```python
from build123d import *

# Parameters (mm, degrees)
SKETCH1_W           = 25
SKETCH1_H           = 50
BOSS_EXTRUDE1_DEPTH = 4.5
CUT_EXTRUDE1_DEPTH  = 4.5
LPATTERN1_COUNT     = 2
LPATTERN1_PITCH     = 16
CUT_EXTRUDE2_REACH  = 6.5


with BuildPart() as part:
    # Sketch1 → Boss-Extrude1 (new body)
    with BuildSketch(Plane.XY):
        with Locations((12.5, 25)):
            Rectangle(SKETCH1_W, SKETCH1_H)
    extrude(amount=BOSS_EXTRUDE1_DEPTH)

    # Sketch2 → Cut-Extrude1 (cut)
    with BuildSketch(Plane.XY.offset(4.5)):
        with BuildLine():
            Line((12.5, 10.25), (14.25, 10.25))
            ThreePointArc((14.25, 10.25), (14.636370331, 9.953527618), (14.45, 9.503589838))
            ThreePointArc((14.45, 9.503589838), (14.303589838, 9.357179677), (14.25, 9.157179677))
            Line((14.25, 9.157179677), (14.25, 8))
            Line((14.25, 8), (14.25, 6.842820323))
            ThreePointArc((14.25, 6.842820323), (14.303589838, 6.642820323), (14.45, 6.496410162))
            ThreePointArc((14.45, 6.496410162), (14.636370331, 6.046472382), (14.25, 5.75))
            Line((14.25, 5.75), (12.5, 5.75))
            Line((12.5, 5.75), (10.75, 5.75))
            ThreePointArc((10.75, 5.75), (10.363629669, 6.046472382), (10.55, 6.496410162))
            ThreePointArc((10.55, 6.496410162), (10.696410162, 6.642820323), (10.75, 6.842820323))
            Line((10.75, 6.842820323), (10.75, 8))
            Line((10.75, 8), (10.75, 9.157179677))
            ThreePointArc((10.75, 9.157179677), (10.696410162, 9.357179677), (10.55, 9.503589838))
            ThreePointArc((10.55, 9.503589838), (10.363629669, 9.953527618), (10.75, 10.25))
            Line((10.75, 10.25), (12.5, 10.25))
        make_face()
    cut_extrude1 = extrude(amount=-CUT_EXTRUDE1_DEPTH, mode=Mode.SUBTRACT)

    # LPattern1: Cut-Extrude1 ×2
    with Locations(*[(0, i * LPATTERN1_PITCH, 0) for i in range(1, LPATTERN1_COUNT)]):
        add(cut_extrude1, mode=Mode.SUBTRACT)

    # Sketch3 → Cut-Extrude2 (cut, up to next)
    with BuildSketch(Plane.XY.offset(4.5), mode=Mode.PRIVATE) as cut_extrude2_sk1:
        with BuildLine():
            Line((6.5, 18.25), (18.5, 18.25))
            ThreePointArc((18.5, 18.25), (18.886370331, 17.953527618), (18.7, 17.503589838))
            ThreePointArc((18.7, 17.503589838), (18.553589838, 17.357179677), (18.5, 17.157179677))
            Line((18.5, 17.157179677), (18.5, 14.842820323))
            ThreePointArc((18.5, 14.842820323), (18.553589838, 14.642820323), (18.7, 14.496410162))
            ThreePointArc((18.7, 14.496410162), (18.886370331, 14.046472382), (18.5, 13.75))
            Line((18.5, 13.75), (6.5, 13.75))
            ThreePointArc((6.5, 13.75), (6.113629669, 14.046472382), (6.3, 14.496410162))
            ThreePointArc((6.3, 14.496410162), (6.446410162, 14.642820323), (6.5, 14.842820323))
            Line((6.5, 14.842820323), (6.5, 17.157179677))
            ThreePointArc((6.5, 17.157179677), (6.446410162, 17.357179677), (6.3, 17.503589838))
            ThreePointArc((6.3, 17.503589838), (6.113629669, 17.953527618), (6.5, 18.25))
        make_face()
    cut_extrude2_tool1 = extrude(cut_extrude2_sk1.sketch, amount=-CUT_EXTRUDE2_REACH, mode=Mode.PRIVATE) & part.part
    add(cut_extrude2_tool1.solids().sort_by_distance((12.5, 16, 4.5))[0], mode=Mode.SUBTRACT)


solid = part.part
```
The model under review builds one solid part; all positions refer to its coordinate system, in mm. A direction names the side the tool comes from. Round coordinates to 2 decimals unless told otherwise and drop trailing zeros. Write each loop counter-clockwise with the first axis right and the second up, starting at its lowest first coordinate (ties: lowest second). Pieces come first, ordered by that corner, then holes.
(1) Wall thickness on L1, parallel to Y at x = 9.75, z = 3.05; L2, parallel to Y at x = 12, z = 2.35; L3, parallel to X at y = 6.5, z = 4.1: over which ranges is each line inside the solid? List them lowest first.
(2) We need section A-A on x = 13. Give the boundary of the cut face in (y, z).
(3) We need section B-B on z = 3.3. Give the number of separate pieces and of enclosed holes in the cut face, and give its area (3 significant figures).
(4) Machinability: for faces 1 (the flat face through (12, 50, 2)), 2 (the flat face through (6.5, 16, 2)), which of the approach directions +Z, -Z, +X, -X, +Y, -Y give a long, thin tool a straight path to every point of the face, cutting with its end or side? Answer none if there is none.
(5) Mouldability with a two-part tool opening along X and no side actions: class faces 3 (the flat face through (12, 0, 2)), 4 (the flat face through (0, 25, 2)), 5 (the flat face through (10.75, 24, 2)) as +X half, -X half, draft (parallel to the pull), parting line (faces both ways), or undercut.
Findings below:
1. L1: y = 0 to 13.75, 18.25 to 50
1. L2: y = 0 to 5.75, 10.25 to 13.75, 18.25 to 21.75, 26.25 to 50
1. L3: x = 0 to 10.56, 14.44 to 25
2. outline: (0, 0) - (5.75, 0) - (5.75, 4.5) - (0, 4.5) - close; (10.25, 0) - (13.75, 0) - (13.75, 4.5) - (10.25, 4.5) - close; (18.25, 0) - (21.75, 0) - (21.75, 4.5) - (18.25, 4.5) - close; (26.25, 0) - (50, 0) - (50, 4.5) - (26.25, 4.5) - close
3. separate pieces: 1
3. enclosed holes: 3
3. area: 1,160 mm2
4. face 1: +Z, -Z, +X, -X, +Y
4. face 2: +Z, -Z
5. face 3: draft
5. face 4: -X half
5. face 5: undercut
